from build123d import *

# Parameters (mm, degrees)
F0_R     = 75.953987
F1_DEPTH = 9.525
F3_DEPTH = 4.7498
F4_R     = 7.466326
F5_DEPTH = 9.525


with BuildPart() as f1:
    # F0 (on Top) → F1 (new body, symmetric)
    with BuildSketch(Plane.XY):
        Circle(F0_R)
    extrude(amount=F1_DEPTH, both=True)

    # F2 (on face) → F3 (cut)
    with BuildSketch(Plane.XY.offset(9.525)):
        with BuildLine():
            Line((-7.454365, -58.986614), (-7.454365, -58.437368))
            ThreePointArc((-7.454365, -58.437368), (-7.459417, -58.711991), (-7.454365, -58.986614))
        make_face()
        with BuildLine():
            Line((-7.454365, 75.587305), (-7.454365, -58.437368))
            Line((-7.454365, -58.437368), (-7.454365, -58.986614))
            ThreePointArc((-7.454365, -58.986614), (0.144244, -66.177054), (7.473236, -58.711991))
            Line((7.473236, -58.711991), (7.473236, 75.585441))
            ThreePointArc((7.473236, 75.585441), (0.009481, 75.953987), (-7.454365, 75.587305))
        make_face()
    extrude(amount=-F3_DEPTH, mode=Mode.SUBTRACT)

    # F4 (on face) → F5 (cut)
    with BuildSketch(Plane.XY.offset(9.525)):
        with Locations((0.006909, -58.711991)):
            Circle(F4_R)
    extrude(amount=-F5_DEPTH, mode=Mode.SUBTRACT)


solid = f1.part
Verification items for the finished model (mm, model axes). A direction names the side the tool comes from. Coordinates: 2 decimals unless noted, no trailing zeros. Order: outer loops, then holes, each group sorted by start corner. A loop starts at its lowest first (then second) coordinate and runs counter-clockwise, first axis right, second up.
Item 1: Depth check by flat-ended pin: pin 1 (2 mm diameter, centred on x = 35, z = 7.5, fed in from +Y); pin 2 (4.5 mm diameter, centred on x = -3, y = -27.5, fed in from +Z); pin 3 (8 mm diameter, centred on x = -50.5, z = -5.5, fed in from +Y); pin 4 (12 mm diameter, centred on x = -3.5, y = -62, fed in from +Z) (3 decimals). Enter the tip coordinate at first touch or a pass-through.
Filled in:
pin 1: stops at y = 67.92
pin 2: stops at z = 4.78
pin 3: stops at y = 60.06
pin 4: stops at z = 9.525
Item 2: Section check C-C, the plane y = -21.5. Enter the section's corners in (x, z) (1 decimal), then the cut area to 3 significant figures.
Filled in:
outline: (-72.8, -9.5) - (72.8, -9.5) - (72.8, 9.5) - (7.5, 9.5) - (7.5, 4.8) - (-7.5, 4.8) - (-7.5, 9.5) - (-72.8, 9.5) - close
area: 2,700 mm2
Item 3: Release check for a two-part mould opening along X. For faces 3 (the face through (-1, 1, -9.525)), 4 (the face through (72.45, 22.81, 0.13)), 5 (the face through (-0.02, -66.18, 7.18)) record: +X half, -X half, draft (parallel to the pull), parting line (faces both ways), or undercut.
Filled in:
face 3: draft
face 4: parting line
face 5: undercut
Item 4: Material ranges on L1, parallel to X at y = 2, z = 8.75; L2, parallel to X at y = -10.5, z = 6; L3, parallel to X at y = 2, z = -0.75, recorded low to high.
Filled in:
L1: x = -75.93 to -7.45, 7.47 to 75.93
L2: x = -75.22 to -7.45, 7.47 to 75.22
L3: x = -75.93 to 75.93
Item 5: Section check A-A, the plane y = 0. Enter the section's corners in (x, z) (3 decimals), then the cut area to 3 significant figures.
Filled in:
outline: (-75.954, -9.525) - (75.954, -9.525) - (75.954, 9.525) - (7.473, 9.525) - (7.473, 4.775) - (-7.454, 4.775) - (-7.454, 9.525) - (-75.954, 9.525) - close
area: 2,820 mm2
Item 6: Section check D-D, the plane x = -63. Enter the section's corners in (y, z) (1 decimal).
Filled in:
outline: (-42.4, -9.5) - (42.4, -9.5) - (42.4, 9.5) - (-42.4, 9.5) - close
Item 7: Access from +Z, -Z, +X, -X, +Y, -Y to the whole of each face (thin tool, end or side, straight path). Record for faces 1 (the face through (0, 22, 4.775)), 2 (the face through (16, 1, 9.525)).
Filled in:
face 1: +Z, +Y
face 2: +Z, +X, -X, +Y, -Y
